from build123d import *

# Parameters (mm, degrees)
SKETCH_1_W          = 30
SKETCH_1_H          = 40
SKETCH_1_R          = 1.25
EXTRUDE_1_DEPTH     = 1
SKETCH_2_W          = 0.8
SKETCH_2_H          = 0.8
EXTRUDE_2_DEPTH     = 10
SKETCH_3_W          = 3
SKETCH_3_H          = 1.5
EXTRUDE_3_DEPTH     = 3
SKETCH_4_W          = 2.462162708
SKETCH_4_H          = 0.766502898
CUT_EXTRUDE_1_DEPTH = 1.5


with BuildPart() as part:
    # 草图1 → 凸台-拉伸1 (new body)
    with BuildSketch(Plane.XY):
        Rectangle(SKETCH_1_W, SKETCH_1_H)
        with Locations((-12, 17.25)):
            Circle(SKETCH_1_R, mode=Mode.SUBTRACT)
        with Locations((12, 17.25)):
            Circle(SKETCH_1_R, mode=Mode.SUBTRACT)
        with Locations((12, -17.25)):
            Circle(SKETCH_1_R, mode=Mode.SUBTRACT)
        with Locations((-12, -17.25)):
            Circle(SKETCH_1_R, mode=Mode.SUBTRACT)
    extrude(amount=EXTRUDE_1_DEPTH)

    # 草图2 → 凸台-拉伸2 (add)
    with BuildSketch(Plane.XY.offset(1)):
        with Locations((-12, -10)):
            Rectangle(SKETCH_2_W, SKETCH_2_H)
        with Locations((-12, -12)):
            Rectangle(SKETCH_2_W, SKETCH_2_H)
        with Locations((-12, -8)):
            Rectangle(SKETCH_2_W, SKETCH_2_H)
        with Locations((-12, -6)):
            Rectangle(SKETCH_2_W, SKETCH_2_H)
        with Locations((-12, -4)):
            Rectangle(SKETCH_2_W, SKETCH_2_H)
        with Locations((-12, -2)):
            Rectangle(SKETCH_2_W, SKETCH_2_H)
        with Locations((-12, 0)):
            Rectangle(SKETCH_2_W, SKETCH_2_H)
        with Locations((-12, 2)):
            Rectangle(SKETCH_2_W, SKETCH_2_H)
        with Locations((-12, 4)):
            Rectangle(SKETCH_2_W, SKETCH_2_H)
        with Locations((-12, 6)):
            Rectangle(SKETCH_2_W, SKETCH_2_H)
        with Locations((-12, 8)):
            Rectangle(SKETCH_2_W, SKETCH_2_H)
        with Locations((-12, 10)):
            Rectangle(SKETCH_2_W, SKETCH_2_H)
        with Locations((-10, -10)):
            Rectangle(SKETCH_2_W, SKETCH_2_H)
        with Locations((-10, -12)):
            Rectangle(SKETCH_2_W, SKETCH_2_H)
        with Locations((-10, -8)):
            Rectangle(SKETCH_2_W, SKETCH_2_H)
        with Locations((-10, -6)):
            Rectangle(SKETCH_2_W, SKETCH_2_H)
        with Locations((-10, -4)):
            Rectangle(SKETCH_2_W, SKETCH_2_H)
        with Locations((-10, -2)):
            Rectangle(SKETCH_2_W, SKETCH_2_H)
        with Locations((-10, 0)):
            Rectangle(SKETCH_2_W, SKETCH_2_H)
        with Locations((-10, 2)):
            Rectangle(SKETCH_2_W, SKETCH_2_H)
        with Locations((-10, 4)):
            Rectangle(SKETCH_2_W, SKETCH_2_H)
        with Locations((-10, 6)):
            Rectangle(SKETCH_2_W, SKETCH_2_H)
        with Locations((-10, 8)):
            Rectangle(SKETCH_2_W, SKETCH_2_H)
        with Locations((-10, 10)):
            Rectangle(SKETCH_2_W, SKETCH_2_H)
        with Locations((-8, -10)):
            Rectangle(SKETCH_2_W, SKETCH_2_H)
        with Locations((-8, -12)):
            Rectangle(SKETCH_2_W, SKETCH_2_H)
        with Locations((-8, -8)):
            Rectangle(SKETCH_2_W, SKETCH_2_H)
        with Locations((-8, -6)):
            Rectangle(SKETCH_2_W, SKETCH_2_H)
        with Locations((-8, -4)):
            Rectangle(SKETCH_2_W, SKETCH_2_H)
        with Locations((-8, -2)):
            Rectangle(SKETCH_2_W, SKETCH_2_H)
        with Locations((-8, 0)):
            Rectangle(SKETCH_2_W, SKETCH_2_H)
        with Locations((-8, 2)):
            Rectangle(SKETCH_2_W, SKETCH_2_H)
        with Locations((-8, 4)):
            Rectangle(SKETCH_2_W, SKETCH_2_H)
        with Locations((-8, 6)):
            Rectangle(SKETCH_2_W, SKETCH_2_H)
        with Locations((-8, 8)):
            Rectangle(SKETCH_2_W, SKETCH_2_H)
        with Locations((-8, 10)):
            Rectangle(SKETCH_2_W, SKETCH_2_H)
    extrude(amount=EXTRUDE_2_DEPTH)

    # 草图3 → 凸台-拉伸3 (add)
    with BuildSketch(Plane(origin=(0, 20, 0), x_dir=(1, 0, 0), z_dir=(0, 1, 0))):
        with Locations((0, -1.75)):
            Rectangle(SKETCH_3_W, SKETCH_3_H)
    extrude(amount=-EXTRUDE_3_DEPTH)

    # 草图4 → 切除-拉伸1 (cut)
    with BuildSketch(Plane(origin=(0, 20, 0), x_dir=(1, 0, 0), z_dir=(0, 1, 0))):
        with Locations((0, -1.75)):
            Rectangle(SKETCH_4_W, SKETCH_4_H)
    extrude(amount=-CUT_EXTRUDE_1_DEPTH, mode=Mode.SUBTRACT)


solid = part.part
Read the model definition and answer for the solid it produces. Units are mm, in the model's axes. A direction names the side the tool comes from. Round coordinates to 2 decimals unless told otherwise and drop trailing zeros. Write each loop counter-clockwise with the first axis right and the second up, starting at its lowest first coordinate (ties: lowest second). Pieces come first, ordered by that corner, then holes.
1. The part is cut by section C-C, the plane z = 6.5. State how many separate pieces and enclosed holes the cut face has, then the cut area to 3 significant figures.
2. The part is cut by section A-A, the plane y = -17.25. Determine the outline of the cut face in (x, z).
3. Determine the mould class of faces 6 (the face through (-10, -12.4, 6)), 7 (the face through (-8, -10.4, 6)), 8 (the face through (-12, 10.4, 6)), 9 (the face through (0, 19, 2.133)) for opening direction Y: pulls with the +Y half, pulls with the -Y half, needs draft (parallel to the pull), parting line crosses it, or undercut.
4. Given pin 1 Ø0.6 at (y, z) = (-2, 7.5) entering from -X; pin 2 Ø4 at (x, y) = (-1, 10) entering from +Z; pin 3 Ø3 at (y, z) = (-15.5, 6.5) entering from -X; pin 4 Ø0.9 at (x, z) = (-12, 5.5) entering from -Y, each flat-ended and moving along its own axis, determine where each tip first touches the part or whether it passes through.
5. Which of the six approach directions +Z, -Z, +X, -X, +Y, -Y give full straight-line access (tool end or side, diameter ignored) to faces 1 (the face through (-12, 0.4, 6)), 2 (the face through (11.079, 18.095, 0.493)), 3 (the face through (-10, -10, 11)), 4 (the face through (1.5, 19, 2)), 5 (the face through (-11.6, -10, 6))?
6. The part is cut by section B-B, the plane x = 12. Determine the outline of the cut face in (y, z).
7. Straight lines are drawn through the part: L1, parallel to Y at x = -12, z = 0.65; L2, parallel to Z at x = 8.5, y = -18. For each, find the intervals that lie inside material, in ascending order.
8. The part is cut by section D-D, the plane x = 5.75. Determine the outline of the cut face in (y, z), then the cut area to 3 significant figures.
Values:
1. separate pieces: 36
1. enclosed holes: 0
1. area: 23.0 mm2
2. outline: (-15, 0) - (-13.25, 0) - (-13.25, 1) - (-15, 1) - close; (-10.75, 0) - (10.75, 0) - (10.75, 1) - (-10.75, 1) - close; (13.25, 0) - (15, 0) - (15, 1) - (13.25, 1) - close
3. face 6: pulls with the -Y half
3. face 7: undercut
3. face 8: pulls with the +Y half
3. face 9: needs draft
4. pin 1: stops at x = -12.4
4. pin 2: stops at z = 1
4. pin 3: passes through
4. pin 4: stops at y = -12.4
5. face 1: +Z, +X, -X
5. face 2: +Z, -Z
5. face 3: +Z, +X, -X, +Y, -Y
5. face 4: +Z, +X, +Y, -Y
5. face 5: +Z, +Y, -Y
6. outline: (-20, 0) - (-18.5, 0) - (-18.5, 1) - (-20, 1) - close; (-16, 0) - (16, 0) - (16, 1) - (-16, 1) - close; (18.5, 0) - (20, 0) - (20, 1) - (18.5, 1) - close
7. L1: y = -20 to -18.5, -16 to 16, 18.5 to 20
7. L2: z = 0 to 1
8. outline: (-20, 0) - (20, 0) - (20, 1) - (-20, 1) - close
8. area: 40.0 mm2
